Source: CAD feature listing. Evaluate the final solid. Frame: model axes, mm. Face numbers are marked on the shaded views. Round coordinates to 2 decimals unless told otherwise and drop trailing zeros. Write each loop counter-clockwise with the first axis right and the second up, starting at its lowest first coordinate (ties: lowest second). Pieces come first, ordered by that corner, then holes. Notation, with made-up numbers: M -6.75,25.25 L 33.25,25.25 A22 ccw 33.25,46.25 Z; hole C 14,45 d10. An arc over 180 degrees is marked long. Use a Markdown table: item, result.
```python
from build123d import *

# Parameters (mm, degrees)
SKETCH1_W          = 50.8
SKETCH1_H          = 381
BASE_EXTRUDE_DEPTH = 12.7
SKETCH2_R          = 3.175
CUT_EXTRUDE1_DEPTH = 193.605036279
CHAMFER1_SIZE      = 3.175
FILLET1_R          = 6.35
FILLET2_R          = 3.048
SHELL1_T           = -1.524
RIB1_REACH         = 194.511
SKETCH3_WALLS_W    = 1.524
SKETCH3_WALLS_H    = 717.22110579
RIB1_DRAFT_ANGLE   = 3
FILLET3_R          = 0.80298
FILLET4_R          = 0.762
FILLET5_R          = 2.54


with BuildPart() as part:
    # Sketch1 → Base-Extrude (new body)
    with BuildSketch(Plane.XY):
        Rectangle(SKETCH1_W, SKETCH1_H)
    extrude(amount=BASE_EXTRUDE_DEPTH)

    # Sketch2 → Cut-Extrude1 (cut, through all)
    with BuildSketch(Plane.XY.offset(12.7)):
        with Locations((0, -165.1)):
            Circle(SKETCH2_R)
        with Locations((0, 165.1)):
            Circle(SKETCH2_R)
    extrude(amount=-CUT_EXTRUDE1_DEPTH, mode=Mode.SUBTRACT)

    # Chamfer1
    chamfer1_edges = [part.edges().sort_by_distance(p)[0] for p in [
        (-3.175, -165.1, 12.7),
        (-3.175, 165.1, 12.7),
    ]]
    chamfer(chamfer1_edges, length=CHAMFER1_SIZE)

    # Fillet1
    fillet1_edges = [part.edges().sort_by_distance(p)[0] for p in [
        (25.4, -190.5, 6.35),
        (-25.4, -190.5, 6.35),
        (-25.4, 190.5, 6.35),
        (25.4, 190.5, 6.35),
    ]]
    fillet(fillet1_edges, radius=FILLET1_R)

    # Fillet2
    fillet2_edges = [part.edges().sort_by_distance(p)[0] for p in [
        (25.4, 0, 12.7),
        (0, -190.5, 12.7),
        (0, 190.5, 12.7),
        (-25.4, 0, 12.7),
        (23.540128061, 188.640128061, 12.7),
        (-23.540128061, 188.640128061, 12.7),
        (-23.540128061, -188.640128061, 12.7),
        (23.540128061, -188.640128061, 12.7),
    ]]
    fillet(fillet2_edges, radius=FILLET2_R)

    # Shell1
    shell1_openings = [part.faces().sort_by_distance(p)[0] for p in [
        (0, 0, 0),
    ]]
    offset(amount=SHELL1_T, openings=shell1_openings, kind=Kind.INTERSECTION)

    # Sketch3 walls → Rib1 (add, up to next)
    with BuildSketch(Plane(origin=(0, 0, 1.524), x_dir=(-1, 0, 0), z_dir=(0, 0, -1)), mode=Mode.PRIVATE) as rib1_sk1:
        Rectangle(SKETCH3_WALLS_W, SKETCH3_WALLS_H)
    rib1_tool1 = extrude(rib1_sk1.sketch, amount=-RIB1_REACH, mode=Mode.PRIVATE) - part.part
    add(rib1_tool1.solids().sort_by_distance((0, 0, 1.524))[0])

    # Rib1 draft
    rib1_draft_faces = [part.faces().sort_by_distance(p)[0] for p in [
        (0.762, 0, 1.905),
        (-0.762, 0, 1.905),
    ]]
    draft(rib1_draft_faces, Plane(origin=(0, 0, 1.524), x_dir=(-1, 0, 0), z_dir=(0, 0, -1)), RIB1_DRAFT_ANGLE)

    # Fillet3
    fillet3_edges = [part.edges().sort_by_distance(p)[0] for p in [
        (0.762, 0, 1.524),
        (-0.762, 0, 1.524),
    ]]
    fillet(fillet3_edges, radius=FILLET3_R - 0.0001)  # a hair under: the kernel refuses the full size

    # Fillet4
    fillet4_edges = [part.edges().sort_by_distance(p)[0] for p in [
        (25.4, 0, 0),
        (0, -190.5, 0),
        (-25.4, 0, 0),
        (0, 190.5, 0),
        (23.540128061, 188.640128061, 0),
        (-23.540128061, 188.640128061, 0),
        (-23.540128061, -188.640128061, 0),
        (23.540128061, -188.640128061, 0),
        (23.876, 0, 0),
        (-23.876, 0, 0),
        (0, -188.976, 0),
        (0, 188.976, 0),
    ]]
    fillet(fillet4_edges, radius=FILLET4_R - 0.0001)  # a hair under: the kernel refuses the full size

    # Fillet5
    fillet5_edges = [part.edges().sort_by_distance(p)[0] for p in [
        (-2.888343865, -168.80649035, 8.893738531),
        (-2.888343865, 168.80649035, 8.893738531),
    ]]
    fillet(fillet5_edges, radius=FILLET5_R)


solid = part.part
```
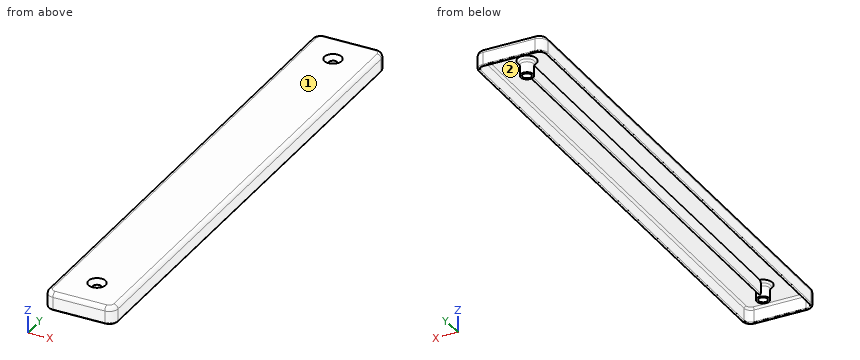
Q1. Section A-A on z = 4.5. Return loops of the section in (x, y) (3 decimals).
Results are:
| item | result |
|---|---|
| outline | M -25.4,-184.15 A6.35 ccw -19.05,-190.5 L 19.05,-190.5 A6.35 ccw 25.4,-184.15 L 25.4,184.15 A6.35 ccw 19.05,190.5 L -19.05,190.5 A6.35 ccw -25.4,184.15 Z; M -0.918,-160.492 A4.699 ccw long 0.918,-160.492 L 0.918,160.492 A4.699 ccw long -0.918,160.492 Z; hole M -23.876,-184.15 A4.826 ccw -19.05,-188.976 L 19.05,-188.976 A4.826 ccw 23.876,-184.15 L 23.876,184.15 A4.826 ccw 19.05,188.976 L -19.05,188.976 A4.826 ccw -23.876,184.15 Z; hole C 0,-165.1 d6.35; hole C 0,165.1 d6.35 |
Q2. Mould query, pull axis Y, two halves, no side actions, for the marked faces 1 and 2. Classes: +Y half, -Y half, draft (parallel to the pull), parting line (faces both ways), or undercut.
Results are:
| item | result |
|---|---|
| face 1 | draft |
| face 2 | undercut |
Q3. First-contact query: pin 1 Ø7.5 at (x, y) = (0, 165.1) entering from +Z; pin 2 Ø4 at (x, y) = (2, -147.5) entering from -Z. Flat tips, straight axial feed; report the tip coordinate or a pass-through.
Results are:
| item | result |
|---|---|
| pin 1 | z = 10.1 |
| pin 2 | z = 1.52 |
Q4. Line query: L1, parallel to X at y = -108, z = 2.5; L2, parallel to X at y = 165.1, z = 5.5 (3 decimals); L3, parallel to Y at x = 0, z = 4.5 (3 decimals). Output: solid intervals per line, ascending.
Results are:
| item | result |
|---|---|
| L1 | -25.4 to -23.88, -0.81 to 0.81, 23.88 to 25.4 |
| L2 | -25.4 to -23.876, -4.699 to -3.175, 3.175 to 4.699, 23.876 to 25.4 |
| L3 | -190.5 to -188.976, -169.799 to -168.275, -161.925 to 161.925, 168.275 to 169.799, 188.976 to 190.5 |
